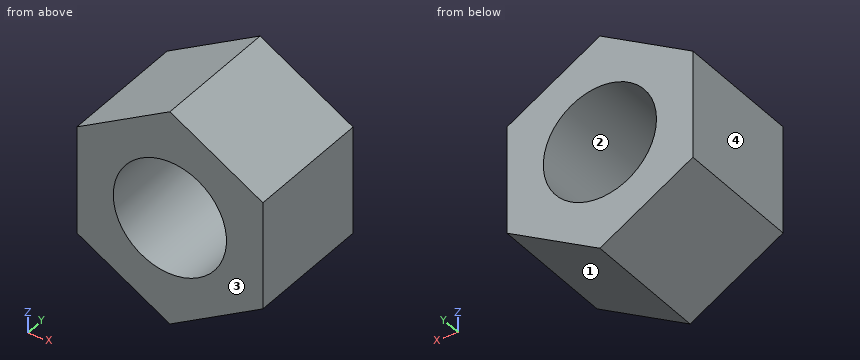
```python
from build123d import *

# Parameters (mm, degrees)
F1_DEPTH = 25.4
F3_D     = 22.225


with BuildPart() as f1:
    # F0 (on Front) → F1 (new body)
    with BuildSketch(Plane.XZ):
        Polygon((18.25625, -10.540251), (18.25625, 10.540251), (0, 21.080502), (-18.25625, 10.540251), (-18.25625, -10.540251), (0, -21.080502), align=None)
    extrude(amount=F1_DEPTH)

    # F3 (through all)
    with Locations(Plane.XZ.offset(25.4)):
        with Locations((0, 0)):
            Hole(F3_D / 2)


solid = f1.part
```
Geometry check sheet. Reference: the model listing, model coordinates, mm. Face numbers are marked on the shaded views. Give positions to 0.01 mm unless a question says otherwise; leave off trailing zeros. Write each loop counter-clockwise with the first axis right and the second up, starting at its lowest first coordinate (ties: lowest second). Pieces come first, ordered by that corner, then holes. Notation, with made-up numbers: (-29.75, 72.5) -> (12.25, 72.5) arc R32 cw to (12.25, 101.5) -> close; hole circle Ø11 at (-11.75, -21). An arc over 180 degrees is marked (long way). Use one line per item in the form item = value.
Item 1: Depth check by flat-ended pin: pin 1 Ø1.5 at (x, z) = (14.5, -5) entering from +Y; pin 2 Ø1 at (x, y) = (-6.5, -6.5) entering from +Z; pin 3 Ø6 at (x, y) = (-4, -12.5) entering from -Z. Enter the tip coordinate at first touch or a pass-through.
Results list:
pin_1 = 0
pin_2 = 17.62
pin_3 = -20.5
Item 2: Sectioned sample at B-B on x = 9. Enter the section's corners in (y, z).
Results list:
outline = (-25.4, -15.88) -> (0, -15.88) -> (0, -6.52) -> (-25.4, -6.52) -> close; (-25.4, 6.52) -> (0, 6.52) -> (0, 15.88) -> (-25.4, 15.88) -> close
Item 3: Scan lines: line 1 (Z direction, x = 0, y = -18.5); line 2 (X direction, y = -19.25, z = 3.5); line 3 (Z direction, x = 7.5, y = -24). Record each from-to range of solid material in increasing order.
Results list:
line_1 = -21.08 to -11.11, 11.11 to 21.08
line_2 = -18.26 to -10.55, 10.55 to 18.26
line_3 = -16.75 to -8.2, 8.2 to 16.75
Item 4: Mould release check, pull along X, two halves, no side actions. Record for the marked faces 1, 2, 3 and 4: released by +X, released by -X, zero draft, split by the parting line, or undercut.
Results list:
face_1 = released by +X
face_2 = undercut
face_3 = zero draft
face_4 = released by -X
Item 5: Sectioned sample at C-C on y = -8. Enter the section's corners in (x, z) (1 decimal).
Results list:
outline = (-18.3, -10.5) -> (0, -21.1) -> (18.3, -10.5) -> (18.3, 10.5) -> (0, 21.1) -> (-18.3, 10.5) -> close; hole circle Ø22.2 at (0, 0)
Item 6: Sectioned sample at D-D on z = -13.5. Enter the section's corners in (x, y), plus the area to 3 significant figures.
Results list:
outline = (-13.13, -25.4) -> (13.13, -25.4) -> (13.13, 0) -> (-13.13, 0) -> close
area = 667 mm2
Item 7: Sectioned sample at A-A on z = 0. Enter the section's corners in (x, y), plus the area to 3 significant figures.
Results list:
outline = (-18.26, -25.4) -> (-11.11, -25.4) -> (-11.11, 0) -> (-18.26, 0) -> close; (11.11, -25.4) -> (18.26, -25.4) -> (18.26, 0) -> (11.11, 0) -> close
area = 363 mm2
